```python
from build123d import *

# Parameters (mm, degrees)
BOSS_EXTRUDE1_DEPTH = 3.2
SKETCH2_R           = 2.4
BOSS_EXTRUDE2_DEPTH = 1.8
SKETCH3_W           = 4.8
SKETCH3_H           = 4.8
CUT_EXTRUDE1_DEPTH  = 1.8


with BuildPart() as part:
    # Sketch1 → Boss-Extrude1 (new body)
    with BuildSketch(Plane(origin=(0, 0, 0), x_dir=(1, 0, 0), z_dir=(0, 1, 0))):
        with BuildLine():
            Line((0, 2.4), (-1.5, 2.4))
            ThreePointArc((-1.5, 2.4), (-2.704535849, 1.312504512), (-4.299182736, 1.011415906))
            ThreePointArc((-4.299182736, 1.011415906), (-4.980961953, 1.823928736), (-4.168449122, 2.505707953))
            ThreePointArc((-4.168449122, 2.505707953), (-2.537715508, 4), (-4.168449122, 5.494292047))
            ThreePointArc((-4.168449122, 5.494292047), (-4.980961953, 6.176071264), (-4.299182736, 6.988584094))
            ThreePointArc((-4.299182736, 6.988584094), (-2.704535849, 6.687495488), (-1.5, 5.6))
            Line((-1.5, 5.6), (0, 5.6))
            Line((0, 5.6), (0, 8))
            Line((0, 8), (8, 8))
            Line((8, 8), (8, 0))
            Line((8, 0), (0, 0))
            Line((0, 0), (0, 2.4))
        make_face()
    extrude(amount=BOSS_EXTRUDE1_DEPTH)

    # Sketch2 → Boss-Extrude2 (add)
    with BuildSketch(Plane(origin=(0, 3.2, 0), x_dir=(1, 0, 0), z_dir=(0, 1, 0))):
        with Locations(Location((4, 4, 0), (0, 0, 270))):
            Circle(SKETCH2_R)
    extrude(amount=BOSS_EXTRUDE2_DEPTH)

    # Sketch3 → Cut-Extrude1 (cut)
    with BuildSketch(Plane.XZ):
        with Locations((4, -4)):
            Rectangle(SKETCH3_W, SKETCH3_H)
    extrude(amount=-CUT_EXTRUDE1_DEPTH, mode=Mode.SUBTRACT)


solid = part.part
```
The listing builds one solid part. Answer for the finished solid, in the listing's coordinates (mm). A direction names the side the tool comes from. Coordinates: 2 decimals unless noted, no trailing zeros. Loops run counter-clockwise (first coordinate to the right, second up) from the corner with the lowest first, then second, coordinate; pieces in that order, holes last. Notation, with made-up numbers: (21.25, 89) -> (67.25, 89) arc R18 cw to (67.25, 95) -> close; hole circle Ø10 at (3.25, -3). An arc over 180 degrees is marked (long way). Use one line per item in the form item = value. Start each with the question number.
Item 1: A tool of negligible diameter and unlimited length cuts with its end or side. For faces 4 (the face through (1.6, 1, -4)), 5 (the face through (-1, 2, -2.4)), 6 (the face through (0, 2, -7)), 7 (the face through (6.024, 4.087, -2.71)), from which of +Z, -Z, +X, -X, +Y, -Y can it reach the whole face along a straight path? Write none if from no direction.
Item 2: The part is cut by section B-B on z = -6.25. Determine the outline of the cut face in (x, y), then the cut area to 3 significant figures.
Item 3: The part is cut by section C-C on y = 0.75. Determine the outline of the cut face in (x, z).
Item 4: The part is cut by section A-A on x = 4. Determine the outline of the cut face in (y, z), then the cut area to 3 significant figures.
Item 5: The part is cut by section D-D on z = -4. Determine the outline of the cut face in (x, y), then the cut area to 3 significant figures.
Item 6: Flat-ended cylindrical pins translate along their axes: pin 1 Ø3.5 at (x, z) = (-4.04, -4) entering from +Y; pin 2 Ø0.5 at (y, z) = (1, -5) entering from -X; pin 3 Ø1.4 at (x, z) = (4, -5) entering from -Y. Find the tip coordinate at first contact, or state that the pin passes through.
Item 7: The mould has two halves that part along Z. Classify faces 1 (the face through (4, 1.8, -4)), 2 (the face through (1.6, 3.2, -4.9)), 3 (the face through (-1, 2, -5.6)): released by +Z, released by -Z, zero draft, split by the parting line, or undercut.
Item 8: Consider L1, parallel to X at y = 1, z = -4; L2, parallel to Z at x = 2.25, y = 0.85; L3, parallel to Y at x = 3, z = -2. Determine where each line is inside the solid, lowest interval first. Write a range as [from, to].
Answer key:
q1.face_4 = -Y
q1.face_5 = +Z, +Y, -Y
q1.face_6 = -Z, +Y, -Y
q1.face_7 = +Y
q2.outline = (-4.98, 0) -> (-2.05, 0) -> (-2.05, 3.2) -> (-4.98, 3.2) -> close; (0, 0) -> (1.6, 0) -> (1.6, 1.8) -> (6.4, 1.8) -> (6.4, 0) -> (8, 0) -> (8, 3.2) -> (4.84, 3.2) -> (4.84, 5) -> (3.16, 5) -> (3.16, 3.2) -> (0, 3.2) -> close
q2.area = 29.3 mm2
q3.outline = (-4.3, -6.99) arc R3 ccw to (-1.5, -5.6) -> (0, -5.6) -> (0, -8) -> (8, -8) -> (8, 0) -> (0, 0) -> (0, -2.4) -> (-1.5, -2.4) arc R3 ccw to (-4.3, -1.01) arc R0.75 ccw to (-4.17, -2.51) arc R1.5 cw (long way) to (-4.17, -5.49) arc R0.75 ccw to start; hole (1.6, -6.4) -> (6.4, -6.4) -> (6.4, -1.6) -> (1.6, -1.6) -> close
q4.outline = (0, -8) -> (3.2, -8) -> (3.2, -6.4) -> (5, -6.4) -> (5, -1.6) -> (3.2, -1.6) -> (3.2, 0) -> (0, 0) -> (0, -1.6) -> (1.8, -1.6) -> (1.8, -6.4) -> (0, -6.4) -> close
q4.area = 25.6 mm2
q5.outline = (-2.54, 0) -> (1.6, 0) -> (1.6, 1.8) -> (6.4, 1.8) -> (6.4, 0) -> (8, 0) -> (8, 3.2) -> (6.4, 3.2) -> (6.4, 5) -> (1.6, 5) -> (1.6, 3.2) -> (-2.54, 3.2) -> close
q5.area = 33.7 mm2
q6.pin_1 = 3.2
q6.pin_2 = -3.21
q6.pin_3 = 1.8
q7.face_1 = undercut
q7.face_2 = zero draft
q7.face_3 = released by -Z
q8.L1 = [-2.54, 1.6], [6.4, 8]
q8.L2 = [-8, -6.4], [-1.6, 0]
q8.L3 = [1.8, 5]
